```python
from build123d import *

# Parameters (mm, degrees)
CHAMFER_SIZE         = 3
CHAMFER001_SIZE      = 2
BODY_PLACEMENT_ANGLE = 180


with BuildPart() as part:
    # Sketch → Revolution (revolve)
    with BuildSketch(Plane.XZ):
        Polygon((24, 0), (7, 0), (7, 3), (12.5, 3), (12.5, 73), (25, 73), (25, 71), (24, 70), (24, 65), (15.5, 56.5), (15.5, 5), (24, 5), align=None)
    revolve(axis=Axis((0, 0, 0), (0, 0, 1)))

    # Chamfer
    chamfer_edges = [part.edges().sort_by_distance(p)[0] for p in [
        (-12.5, 0, 73),
    ]]
    chamfer(chamfer_edges, length=CHAMFER_SIZE)

    # Chamfer001
    chamfer001_edges = [part.edges().sort_by_distance(p)[0] for p in [
        (-24, 0, 0),
    ]]
    chamfer(chamfer001_edges, length=CHAMFER001_SIZE)


with BuildPart() as part_1:
    # Body placement: moved
    add(part.part.moved(Location((0, 0, -33))).rotate(Axis((0, 0, -33), (0, 1, 0)), BODY_PLACEMENT_ANGLE))


solid = part_1.part
```
CAD build for the part. Positions are in the model's coordinates, mm. A direction names the side the tool comes from. Round coordinates to 2 decimals unless told otherwise and drop trailing zeros. Write each loop counter-clockwise with the first axis right and the second up, starting at its lowest first coordinate (ties: lowest second). Pieces come first, ordered by that corner, then holes. Notation, with made-up numbers: (41, 2) - (76, 2) arc R20 ccw to (76, 36) - close; hole circle Ø2 at (24.25, -26). An arc over 180 degrees is marked (long way). Write item = value, one per line. Start each with the question number.
Q1. Band-saw the part on C-C (z = -58.5). Give the cut face in (x, y).
Q2. Probe L1, parallel to Y at x = 0, z = -33.75; L2, parallel to Z at x = 18, y = 8; L3, parallel to Z at x = 9, y = 19. List the from-to ranges inside material, lowest first. Write a range as from..to.
Q3. Band-saw the part on D-D (z = -97). Give the cut face in (x, y), then the cut area to 3 significant figures.
Q4. Mould opens along Y. For faces 5 (the cylindrical face through (19.05, -14.6, -100.46)), 6 (the flat face through (0, -16, -38)), 7 (the cylindrical face through (-11.923, 3.755, -69.969)) say: pulls with the +Y half, pulls with the -Y half, needs draft (parallel to the pull), parting line crosses it, or undercut.
Q5. Drop flat-ended pins along their axis: pin 1 (1 mm diameter, centred on x = 0.5, z = -98, fed in from -Y); pin 2 (20 mm diameter, centred on x = -3.5, y = 1, fed in from -Z); pin 3 (12 mm diameter, centred on x = -4, z = -70, fed in from +Y). Give the stop position or say it passes through.
Q6. Band-saw the part on A-A (x = 0). Give the cut face in (y, z), then the cut area to 3 significant figures.
Q7. Which spindle directions (+Z, -Z, +X, -X, +Y, -Y) get a long thin tool onto all of the face, cutting with end or side? Do faces 1 (the flat face through (5.4, -5.4, -36)), 2 (the cylindrical face through (23.977, 1.055, -36.479)), 3 (the cylindrical face through (2.018, 15.368, -63.39)), 4 (the flat face through (10.8, 11.5, -106)). Say none if no direction does.
Answers below:
q1.outline = circle Ø31 at (0, 0); hole circle Ø25 at (0, 0)
q2.L1 = -22.75..-7, 7..22.75
q2.L2 = -106..-93.7, -38..-33
q2.L3 = -106..-95.02, -38..-33
q3.outline = circle Ø46 at (0, 0); hole circle Ø25 at (0, 0)
q3.area = 1,170 mm2
q4.face_5 = parting line crosses it
q4.face_6 = needs draft
q4.face_7 = undercut
q5.pin_1 = -24
q5.pin_2 = -104.14
q5.pin_3 = 15.5
q6.outline = (-25, -106) - (-15.5, -106) - (-12.5, -103) - (-12.5, -36) - (-7, -36) - (-7, -33) - (-22, -33) - (-24, -35) - (-24, -38) - (-15.5, -38) - (-15.5, -89.5) - (-24, -98) - (-24, -103) - (-25, -104) - close; (7, -36) - (12.5, -36) - (12.5, -103) - (15.5, -106) - (25, -106) - (25, -104) - (24, -103) - (24, -98) - (15.5, -89.5) - (15.5, -38) - (24, -38) - (24, -35) - (22, -33) - (7, -33) - close
q6.area = 756 mm2
q7.face_1 = -Z
q7.face_2 = +Z
q7.face_3 = none
q7.face_4 = -Z, +X, -X, +Y, -Y
